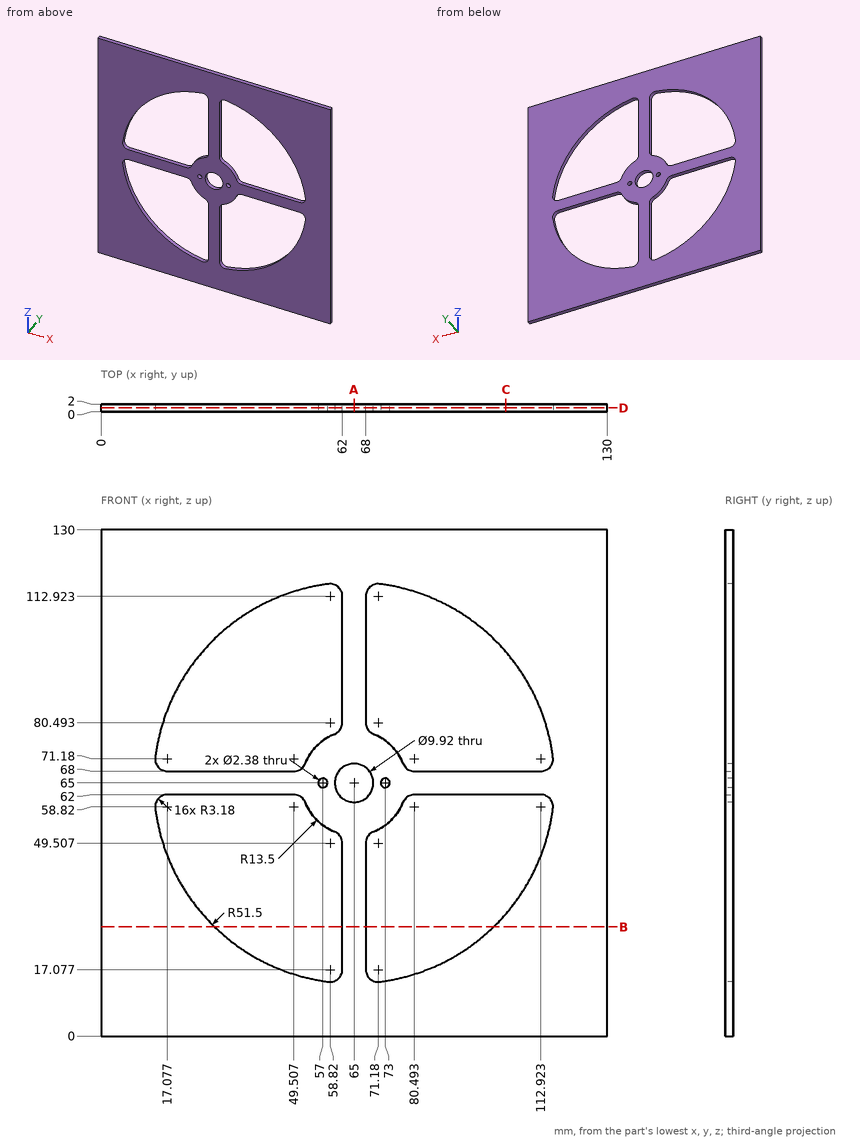
Input: dimensioned drawing with shaded views. Units: mm. Origin: part minimum x, y, z. Give positions to 0.01 mm unless a question says otherwise; leave off trailing zeros. Loops run counter-clockwise (first coordinate to the right, second up) from the corner with the lowest first, then second, coordinate; pieces in that order, holes last. Notation, with made-up numbers: M 6.5,27.25 L 14.5,27.25 A5 ccw 14.5,36.25 Z; hole C 37.25,53 d9. An arc over 180 degrees is marked long. Put each result on its own line as item: value. Start each with the question number.
1) Cut plane C-C (x = 104). Output: boundary loops of the cut face in (y, z).
2) Contact query for a flat-ended pin moving along its axis: pin 1 (3 mm diameter, centred on x = 112.5, z = 52.5, fed in from -Y) (3 decimals). Output: stop coordinate, or through.
3) Cut plane B-B (z = 28). Output: boundary loops of the cut face in (x, y).
4) Ray query, line 1 along Z through (x, y) = (65, 0.8); line 2 along Z through (x, y) = (18, 0.9) (1 decimal); line 3 along Z through (x, y) = (73, 1.3) (1 decimal). Return the intervals inside material, ascending.
5) Cut plane A-A (x = 65). Output: boundary loops of the cut face in (y, z).
6) Cut plane D-D (y = 1). Give the number of separate pieces and of enclosed holes in the cut face, then the cut area to 4 significant figures.
Verdict:
1. outline: M 0,0 L 2,0 L 2,31.37 L 0,31.37 Z; M 0,62 L 2,62 L 2,68 L 0,68 Z; M 0,98.63 L 2,98.63 L 2,130 L 0,130 Z
2. pin 1: through
3. outline: M 0,0 L 29.18,0 L 29.18,2 L 0,2 Z; M 62,0 L 68,0 L 68,2 L 62,2 Z; M 100.82,0 L 130,0 L 130,2 L 100.82,2 Z
4. line 1: 0 to 60.04, 69.96 to 130
4. line 2: 0 to 43.9, 62 to 68, 86.1 to 130
4. line 3: 0 to 14.1, 54.1 to 63.8, 66.2 to 75.9, 115.9 to 130
5. outline: M 0,0 L 2,0 L 2,60.04 L 0,60.04 Z; M 0,69.96 L 2,69.96 L 2,130 L 0,130 Z
6. separate pieces: 1
6. enclosed holes: 7
6. area: 10,000 mm2
